Can you work these out from the model? Positions are in its coordinate system, mm. A direction names the side the tool comes from. Coordinates: 2 decimals unless noted, no trailing zeros. Order: outer loops, then holes, each group sorted by start corner. A loop starts at its lowest first (then second) coordinate and runs counter-clockwise, first axis right, second up. Notation, with made-up numbers: (62.25, -15) -> (74.25, -15) arc R10 ccw to (74.25, -3) -> close; hole circle Ø2 at (35, -33.5). An arc over 180 degrees is marked (long way). Use a Markdown table: item, result. Add a question column.
1. For pin 1 Ø8 at (x, y) = (29.5, 1.5) entering from +Z; pin 2 Ø6 at (x, z) = (29, -2) entering from -Y; pin 3 Ø1.5 at (x, y) = (9.5, -1.5) entering from -Z, each with a flat end and sliding along its axis, tell me the tip position at first contact or that it passes through.
2. If I drill on line 1 along X through (y, z) = (-1.25, -6.5); line 2 along Y through (x, z) = (55, 0.25); line 3 along Z through (x, y) = (0.5, -0.75), over which ranges is the centre line in solid material (lowest first)? Write a range as from..to.
3. Suppose I cut it at A-A, the plane x = 44.5. List the corners of the cut face in (y, z) for me (1 decimal).
4. For faces 1 (the cylindrical face through (50.68, -3.78, -2.9)), 2 (the flat face through (-3.36, -6.15, 3.62)), which set-ups out of +Z, -Z, +X, -X, +Y, -Y let a thin tool reach every point of the face, with its end or its side?
5. Suppose I cut it at B-B, the plane x = 5. List the corners of the cut face in (y, z) for me.
Autodesk Inventor part; units mm, degrees
ref_plane "Work Plane1" through (1.525, 0, 0) normal (0, 0, 1) x (1, 0, 0)
ref_plane "YZ Plane" through (0, 0, 0) normal (1, 0, 0) x (0, 1, 0)
ref_plane "XZ Plane" through (0, 0, 0) normal (0, 1, 0) x (-1, 0, 0)
sketch "Sketch1" plane through (0, 0, 0) normal (0, 0, 1) x (1, 0, 0)
  line L0 (0, 7.1374) -> (0, 4.9276)
  line L1 (25.4, 4.7625) -> (76.2, 4.7625)
  line L2 (76.2, 4.7625) -> (76.2, 0)
  line L3 (76.2, 0) -> (-0.0001, 0)
  line L4 (-15.2401, 0) -> (91.44, 0)
  line L5 (-0.0001, 0) -> (-0.0001, 7.1374)
  line L6 (-0.0001, 7.1374) -> (0, 7.1374)
  line L7 (25.4, 4.7625) -> (21.4311, 4.9276)
  line L8 (21.4311, 4.9276) -> (0, 4.9276)
  line L9 (0, -1.4275) -> (0, 8.5649)
  dimension "d0" = 76.2
  dimension "d1" = 50.8
revolve "Body" add sketch "Sketch1" angle 360 about axis through (76.2, 0, 0) along (-1, 0, 0)
sketch "Sketch2" plane through (-0.0001, 0, 0) normal (-1, 0, 0) x (0, 0, 1)
  line L0 (0, 8.2416) -> (7.1374, 4.1208)
  line L1 (7.1374, 4.1208) -> (7.1374, -4.1208)
  line L2 (7.1374, -4.1208) -> (0, -8.2416)
  line L3 (0, -8.2416) -> (-7.1374, -4.1208)
  line L4 (-7.1374, -4.1208) -> (-7.1374, 4.1208)
  line L5 (-7.1374, 4.1208) -> (0, 8.2416)
  point P0 (0, 0)
  point P1 (0, 0)
  dimension "d11" = 14.2748
extrude "Head" add sketch "Sketch2" along normal blind 6.8072
sketch "Sketch4" plane through (0, 0, 0) normal (0, 0, 1) x (1, 0, 0)
  line L0 (-6.8073, 7.1374) -> (-6.8073, 8.2416)
  line L1 (-6.8073, 8.2416) -> (-6.1698, 8.2416)
  line L2 (-6.1698, 8.2416) -> (-6.8073, 7.1374)
  line L3 (-8.1687, 0) -> (1.3613, 0)
  line L4 (-0.0001, 8.2416) -> (-6.8073, 8.2416)
  line L5 (-6.8073, 4.1208) -> (-6.8073, 8.2416)
  dimension "d5" = 30
  dimension "d19" = 14.2748
revolve "Chamfer1" cut sketch "Sketch4" angle 360 about axis through (-10, 0, 0) along (1, 0, 0)
thread "Thread"
chamfer "Chamfer2" distance 0.9739 distance2 0.9447 1 edges at (76.2, -4.7625, 0) measured on face at (76.2, 1.5414, -0.3799)
ref_plane "Work Plane1" through (1.525, 0, 0) normal (0, 0, 1) x (1, 0, 0)
fillet "Fillet2" radius 0.762 1 edges at (0, -4.9276, 0)
equation "\"d63\" = R"
equation "\"d11\" = SW"
equation "\"d3\" = KOH - SD"
equation "\"d15\" = GEL"
equation "\"d6\" = -0.5 * SPD + 0.5 * GD"
equation "\"d5\" = ANG1"
equation "\"d19\" = SW0"
equation "\"NLG\" = 190.5"
equation "\"GD\" = NND"
equation "\"BDM\" = 9.8552"
equation "\"KOH\" = 6.8072"
equation "\"GEL\" = 31.75"
equation "\"SW\" = 14.2748"
equation "\"SW0\" = SW"
equation "\"SPD\" = GD1"
equation "\"SD2\" = SW"
equation "\"SD\" = 0"
equation "\"ANG1\" = 30deg"
equation "\"GAL\" = 3.96875"
equation "\"GUL\" = 0.238 * GAL"
equation "\"R\" = 0.762"
equation "\"d62\" = -NLG - SD + GUL"
equation "\"GD1\" = 7.5773"
equation "\"THREADDIA\" = 9.525"
equation "\"TOA\" = 30deg"
equation "\"NND\" = 9.525"
equation "\"E0\" = 1.155 * SW"
properties part number "am-1055" material "Steel, Mild"
Worked out:
| question | item | result |
|---|---|---|
| 1 | pin 1 | stops at z = 4.76 |
| 1 | pin 2 | stops at y = -4.76 |
| 1 | pin 3 | stops at z = -4.87 |
| 2 | line 1 | x = -6.81..0 |
| 2 | line 2 | y = -4.76..4.76 |
| 2 | line 3 | z = -4.92..4.92 |
| 3 | outline | circle Ø9.5 at (0, 0) |
| 4 | face 1 | +X |
| 4 | face 2 | +Z, +X, -X, -Y |
| 5 | outline | circle Ø9.86 at (0, 0) |
